Check sheet for the drawn part. Datum: minimum x, y, z corner. Units: mm. Coordinates: 2 decimals unless noted, no trailing zeros. Order: outer loops, then holes, each group sorted by start corner. A loop starts at its lowest first (then second) coordinate and runs counter-clockwise, first axis right, second up. Notation, with made-up numbers: (14, 62) - (27, 62) arc R24 cw to (27, 75) - close; hole circle Ø1 at (-14.5, -35.75). An arc over 180 degrees is marked (long way). Put each result on its own line as item: value.
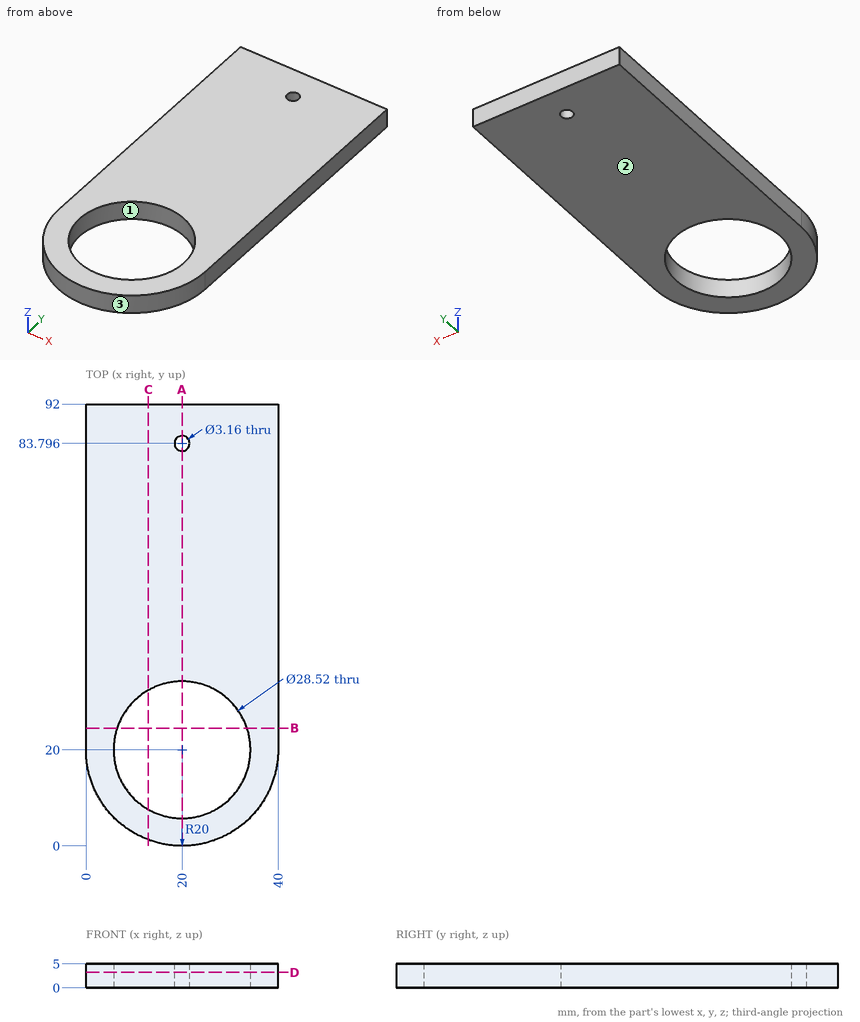
Q1. Section check A-A on x = 20. Record the boundary of the cut face in (y, z).
Answer block:
outline: (0, 0) - (5.74, 0) - (5.74, 5) - (0, 5) - close; (34.26, 0) - (82.22, 0) - (82.22, 5) - (34.26, 5) - close; (85.38, 0) - (92, 0) - (92, 5) - (85.38, 5) - close
Q2. Section check B-B on y = 24.5. Record the boundary of the cut face in (x, z).
Answer block:
outline: (0, 0) - (6.47, 0) - (6.47, 5) - (0, 5) - close; (33.53, 0) - (40, 0) - (40, 5) - (33.53, 5) - close
Q3. Thickness scan on L1, parallel to Y at x = 20, z = 1.25; L2, parallel to X at y = 8.5, z = 0.25; L3, parallel to Y at x = 11, z = 3.1. Record the ranges inside material, lowest first. Write a range as [from, to].
Answer block:
L1: y = [0, 5.74], [34.26, 82.22], [85.38, 92]
L2: x = [3.64, 11.57], [28.43, 36.36]
L3: y = [2.14, 8.94], [31.06, 92]
Q4. Draft check along X on the marked faces 1, 2 and 3. Enter one of: pulls with the +X half, pulls with the -X half, needs draft (parallel to the pull), parting line crosses it, or undercut.
Answer block:
face 1: undercut
face 2: needs draft
face 3: parting line crosses it
Q5. Depth check by flat-ended pin: pin 1 Ø8 at (x, y) = (30, 72.5) entering from -Z; pin 2 Ø2 at (x, z) = (20, 1) entering from -Y. Enter the tip coordinate at first touch or a pass-through.
Answer block:
pin 1: stops at z = 0
pin 2: stops at y = 0
Q6. Section check D-D on z = 3.25. Record the boundary of the cut face in (x, y), then the cut area to 3 significant figures.
Answer block:
outline: (0, 20) arc R20 ccw to (40, 20) - (40, 92) - (0, 92) - close; hole circle Ø28.52 at (20, 20); hole circle Ø3.16 at (20, 83.8)
area: 2,860 mm^2
Q7. Section check C-C on x = 13. Record the boundary of the cut face in (y, z) (1 decimal).
Answer block:
outline: (1.3, 0) - (7.6, 0) - (7.6, 5) - (1.3, 5) - close; (32.4, 0) - (92, 0) - (92, 5) - (32.4, 5) - close
